Geometry check sheet. Reference: the model listing, model coordinates, mm. Face numbers are marked on the shaded views. A direction names the side the tool comes from. Round coordinates to 2 decimals unless told otherwise and drop trailing zeros. Loops run counter-clockwise (first coordinate to the right, second up) from the corner with the lowest first, then second, coordinate; pieces in that order, holes last. Notation, with made-up numbers: M 11.25,-6.75 L 39.25,-6.75 A20 cw 39.25,27.25 Z; hole C -28.75,38 d8. An arc over 180 degrees is marked long. Write item = value, one per line.
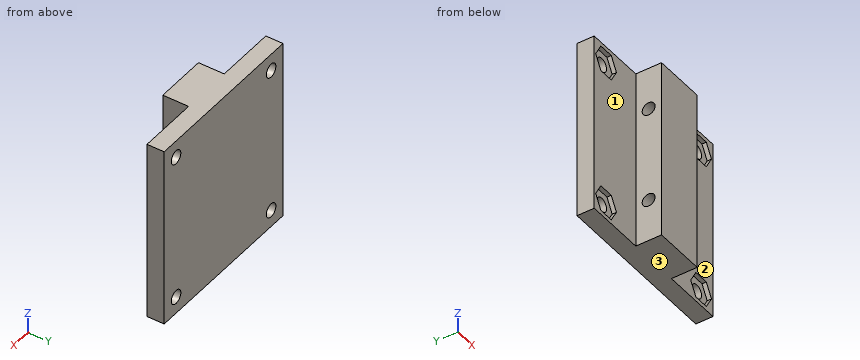
from build123d import *

# Parameters (mm, degrees)
BOSS_EXTRU_1_DEPTH      = 42.5
D_GAGEMENT_M31_D        = 3
D_GAGEMENT_M33_D        = 3.2
ENL_V_MAT_EXTRU_1_DEPTH = 1


with BuildPart() as part:
    # Esquisse1 → Boss.-Extru.1 (new body)
    with BuildSketch(Plane(origin=(0, 0, 0), x_dir=(1, 0, 0), z_dir=(0, 0, -1))):
        Polygon((-1.384510159, -46.220398701), (38.615489841, -46.220398701), (38.615489841, -42.220398701), (24.615489841, -42.220398701), (24.615489841, -36.220398701), (12.615489841, -36.220398701), (12.615489841, -42.220398701), (-1.384510159, -42.220398701), align=None)
    extrude(amount=BOSS_EXTRU_1_DEPTH)

    # Dégagement M31 (through all)
    with Locations(Plane(origin=(24.615489841, 0, 0), x_dir=(0, 0, -1), z_dir=(1, 0, 0))):
        with Locations((10, 39.220398701), (32.5, 39.220398701)):
            Hole(D_GAGEMENT_M31_D / 2)

    # Dégagement M33 (through all)
    with Locations(Plane(origin=(0, 42.220398701, 0), x_dir=(-1, 0, 0), z_dir=(0, -1, 0))):
        with Locations((3, -59.94627318), (-34.615489841, 38.5), (-2.615489841, 38.5), (-2.615489841, 4), (-34.615489841, 4)):
            Hole(D_GAGEMENT_M33_D / 2)

    # Esquisse9 → Enlèv. mat.-Extru.1 (cut)
    with BuildSketch(Plane.XZ.offset(-42.220398701)):
        Polygon((32.865489841, -35.468911087), (31.115489841, -38.5), (32.865489841, -41.531088913), (36.365489841, -41.531088913), (38.115489841, -38.5), (36.365489841, -35.468911087), align=None)
        Polygon((4.365489841, -35.468911087), (0.865489841, -35.468911087), (-0.884510159, -38.5), (0.865489841, -41.531088913), (4.365489841, -41.531088913), (6.115489841, -38.5), align=None)
        Polygon((32.865489841, -0.968911087), (31.115489841, -4), (32.865489841, -7.031088913), (36.365489841, -7.031088913), (38.115489841, -4), (36.365489841, -0.968911087), align=None)
        Polygon((4.365489841, -0.968911087), (0.865489841, -0.968911087), (-0.884510159, -4), (0.865489841, -7.031088913), (4.365489841, -7.031088913), (6.115489841, -4), align=None)
    extrude(amount=-ENL_V_MAT_EXTRU_1_DEPTH, mode=Mode.SUBTRACT)


solid = part.part
(1) Sectioned sample at C-C on x = 35. Record the cut outline in (y, z), then the cut area to 3 significant figures.
Result set:
outline = M 42.22,-42.5 L 46.22,-42.5 L 46.22,-40.05 L 43.22,-40.05 L 43.22,-41.53 L 42.22,-41.53 Z; M 42.22,-35.47 L 43.22,-35.47 L 43.22,-36.95 L 46.22,-36.95 L 46.22,-5.55 L 43.22,-5.55 L 43.22,-7.03 L 42.22,-7.03 Z; M 42.22,-0.97 L 43.22,-0.97 L 43.22,-2.45 L 46.22,-2.45 L 46.22,0 L 42.22,0 Z
area = 139 mm2
(2) Material ranges on line 1 along X through (y, z) = (44.7, -38.5); line 2 along Y through (x, z) = (20.75, -10); line 3 along Z through (x, y) = (31.5, 43), recorded low to high. Write a range as from..to.
Result set:
line_1 = -1.38..1.02, 4.22..33.02, 36.22..38.62
line_2 = 36.22..37.72, 40.72..46.22
line_3 = -42.5..-39.17, -37.83..-4.67, -3.33..0
(3) Sectioned sample at D-D on y = 39.75. Record the cut outline in (x, z), then the cut area to 3 significant figures.
Result set:
outline = M 12.62,-42.5 L 24.62,-42.5 L 24.62,-33.9 L 12.62,-33.9 Z; M 12.62,-31.1 L 24.62,-31.1 L 24.62,-11.4 L 12.62,-11.4 Z; M 12.62,-8.6 L 24.62,-8.6 L 24.62,0 L 12.62,0 Z
area = 443 mm2
(4) Tool access check on the marked faces 1, 2 and 3. Record the directions out of +Z, -Z, +X, -X, +Y, -Y that give a thin tool (end or side, any length) a straight path to the whole face; none if there is none.
Result set:
face_1 = +Z, -Z, -X, -Y
face_2 = +Z, -Z, +X, -Y
face_3 = -Z, +X, -X, +Y, -Y
(5) Depth check by flat-ended pin: pin 1 Ø0.8 at (x, y) = (35.5, 43) entering from +Z; pin 2 Ø1 at (x, z) = (33, -6.5) entering from -Y; pin 3 Ø5 at (y, z) = (39.22, -32.5) entering from -X. Enter the tip coordinate at first touch or a pass-through.
Result set:
pin_1 = 0
pin_2 = 42.22
pin_3 = 12.62
(6) Sectioned sample at A-A on z = -10. Record the cut outline in (x, y), then the cut area to 3 significant figures.
Result set:
outline = M -1.38,42.22 L 12.62,42.22 L 12.62,40.72 L 24.62,40.72 L 24.62,42.22 L 38.62,42.22 L 38.62,46.22 L -1.38,46.22 Z; M 12.62,36.22 L 24.62,36.22 L 24.62,37.72 L 12.62,37.72 Z
area = 196 mm2
(7) Sectioned sample at B-B on y = 45. Record the cut outline in (x, z).
Result set:
outline = M -1.38,-42.5 L 38.62,-42.5 L 38.62,0 L -1.38,0 Z; hole C 2.62,-38.5 d3.2; hole C 2.62,-4 d3.2; hole C 34.62,-38.5 d3.2; hole C 34.62,-4 d3.2
